from build123d import *

# Parameters (mm, degrees)
F1_DEPTH  = 16
F3_DEPTH  = 148
F5_DEPTH  = 148
F6_R      = 3
F7_R      = 3
F8_R      = 1
F9_R      = 1
F11_DEPTH = 10
F13_DEPTH = 10


with BuildPart() as f1:
    # F0 (on Front) → F1 (new body)
    with BuildSketch(Plane.XZ):
        Polygon((130.5555550784, 7), (-19.4444449216, 7), (-19.4444449216, 0), (123.5555550784, 0), (123.5555550784, -143), (130.5555550784, -143), align=None)
    extrude(amount=F1_DEPTH)

    # F2 (on face) → F3 (cut)
    with BuildSketch(Plane(origin=(0, 0, -143), x_dir=(1, 0, 0), z_dir=(0, 0, -1))):
        Polygon((125.5555550784, 10), (123.5555550784, 10), (123.5555550784, 6), (125.5555550784, 6), (125.5555550784, 2), (128.5555550784, 2), (128.5555550784, 14), (125.5555550784, 14), align=None)
    extrude(amount=-F3_DEPTH, mode=Mode.SUBTRACT)

    # F4 (on face) → F5 (cut)
    with BuildSketch(Plane(origin=(-19.4444449216, 0, 0), x_dir=(0, -1, 0), z_dir=(-1, 0, 0))):
        Polygon((6, 2), (6, 0), (10, 0), (10, 2), (14, 2), (14, 5), (2, 5), (2, 2), align=None)
    extrude(amount=-F5_DEPTH, mode=Mode.SUBTRACT)

    # F6
    f6_edges = [f1.edges().sort_by_distance(p)[0] for p in [
        (128.555555, -8, 5),
        (123.555555, -3, 0),
        (123.555555, -13, 0),
    ]]
    fillet(f6_edges, radius=F6_R)

    # F7
    f7_edges = [f1.edges().sort_by_distance(p)[0] for p in [
        (125.555555, -4, 2),
        (125.555555, -12, 2),
    ]]
    fillet(f7_edges, radius=F7_R)

    # F8
    f8_edges = [f1.edges().sort_by_distance(p)[0] for p in [
        (130.555555, -8, 7),
        (55.555555, 0, 7),
        (50.555555, 0, 0),
        (122.676875, 0, -0.87868),
        (-19.444445, 0, 3.5),
        (123.555555, 0, -73),
        (127.055555, 0, -143),
        (130.555555, 0, -68),
    ]]
    fillet(f8_edges, radius=F8_R)

    # F9
    f9_edges = [f1.edges().sort_by_distance(p)[0] for p in [
        (55.055555, -16, 7),
        (130.262662, -16, 6.707107),
        (-19.444445, -16, 3.5),
        (130.555555, -16, -68.5),
        (50.555555, -16, 0),
        (127.055555, -16, -143),
        (122.676875, -16, -0.87868),
        (123.555555, -16, -73),
    ]]
    fillet(f9_edges, radius=F9_R)

    # F10 (on face) → F11 (cut)
    with BuildSketch(Plane(origin=(-19.4444449216, 0, 0), x_dir=(0, -1, 0), z_dir=(-1, 0, 0))):
        Polygon((10, 1), (15, 1), (15, 6), (1, 6), (1, 1), (6, 1), (6, 2), (2, 2), (2, 5), (14, 5), (14, 2), (10, 2), align=None)
    extrude(amount=-F11_DEPTH, mode=Mode.SUBTRACT)

    # F12 (on face) → F13 (cut)
    with BuildSketch(Plane(origin=(0, 0, -143), x_dir=(1, 0, 0), z_dir=(0, 0, -1))):
        Polygon((129.5555550784, 15), (124.5555550784, 15), (124.5555550784, 10), (125.5555550784, 10), (125.5555550784, 14), (128.5555550784, 14), (128.5555550784, 2), (125.5555550784, 2), (125.5555550784, 6), (124.5555550784, 6), (124.5555550784, 1), (129.5555550784, 1), align=None)
    extrude(amount=-F13_DEPTH, mode=Mode.SUBTRACT)


solid = f1.part
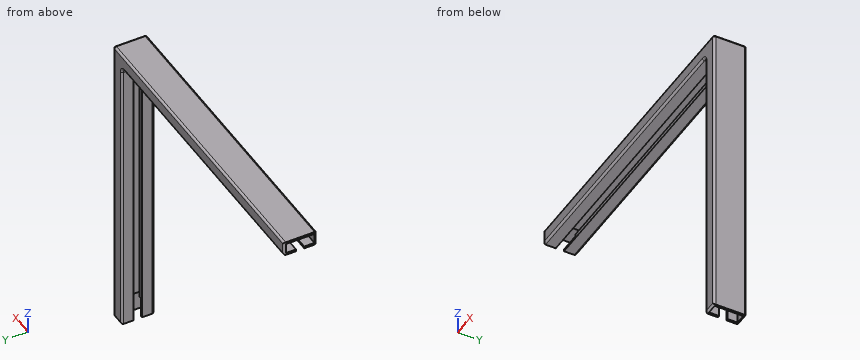
Here's how the part is built. I have some questions about the finished solid (model axes, mm). Round coordinates to 2 decimals unless told otherwise and drop trailing zeros. Order: outer loops, then holes, each group sorted by start corner. A loop starts at its lowest first (then second) coordinate and runs counter-clockwise, first axis right, second up. Notation, with made-up numbers: (-33, 36) -> (12, 36) arc R8 ccw to (12, 51) -> close; hole circle Ø11 at (58.25, -23). An arc over 180 degrees is marked (long way). Return JSON: item names as keys, results as strings.
Q1. For pin 1 Ø5.5 at (y, z) = (-13.5, -51.5) entering from -X; pin 2 Ø5 at (x, y) = (41.5, -6.5) entering from -Z, each with a flat end and sliding along its axis, tell me the tip position at first contact or that it passes through.
Filled sheet:
{"pin 1": "stops at x = 123.56", "pin 2": "stops at z = 0"}
Q2. I need wall thicknesses on line 1 along X through (y, z) = (-2.75, -77.5); line 2 along Z through (x, y) = (1, -3.75); line 3 along Z through (x, y) = (47.5, -9.25). Which ranges of each line are inside material? Lowest first, please. Write a range as from..to.
Filled sheet:
{"line 1": "x = 123.56..125.56, 128.56..130.56", "line 2": "z = 0..2, 5..7", "line 3": "z = 5..7"}
Q3. If we section it at A-A on z = -21: List the corners of the cut face in (x, y) for me, plus the area to 3 significant figures.
Filled sheet:
{"outline": "(123.56, -15) arc R1 ccw to (124.56, -16) -> (129.56, -16) arc R1 ccw to (130.56, -15) -> (130.56, -1) arc R1 ccw to (129.56, 0) -> (124.56, 0) arc R1 ccw to (123.56, -1) -> (123.56, -6) -> (125.56, -6) -> (125.56, -2) -> (128.56, -2) -> (128.56, -14) -> (125.56, -14) -> (125.56, -10) -> (123.56, -10) -> close", "area": "67.1 mm^2"}
Q4. If we section it at B-B on x = 110.5: List the corners of the cut face in (y, z) for me, plus the area to 3 significant figures.
Filled sheet:
{"outline": "(-16, 1) arc R1 ccw to (-15, 0) -> (-10, 0) -> (-10, 2) -> (-14, 2) -> (-14, 5) -> (-2, 5) -> (-2, 2) -> (-6, 2) -> (-6, 0) -> (-1, 0) arc R1 ccw to (0, 1) -> (0, 6) arc R1 ccw to (-1, 7) -> (-15, 7) arc R1 ccw to (-16, 6) -> close", "area": "67.1 mm^2"}
